from build123d import *

# Parameters (mm, degrees)
BOSS_EXTRUDE1_DEPTH = 12
SKETCH3_R           = 3.495
CUT_EXTRUDE2_DEPTH  = 78.961272437
CHAMFER1_SIZE       = 5


with BuildPart() as part:
    # Sketch1 → Boss-Extrude1 (new body)
    with BuildSketch(Plane.XY):
        Polygon((0, 0), (0, 58.6), (-35, 58.6), (-26.195973182, 49.795973182), (-26.195973182, 11.1), (-50, 0), align=None)
    extrude(amount=BOSS_EXTRUDE1_DEPTH)

    # Sketch3 → Cut-Extrude2 (cut, through all)
    with BuildSketch(Plane.XY.offset(12)):
        with Locations((-13.556619589, 25.36)):
            Circle(SKETCH3_R)
    extrude(amount=-CUT_EXTRUDE2_DEPTH, mode=Mode.SUBTRACT)

    # Chamfer1
    chamfer1_edges = [part.edges().sort_by_distance(p)[0] for p in [
        (0, 58.6, 6),
    ]]
    chamfer(chamfer1_edges, length=CHAMFER1_SIZE)


solid = part.part
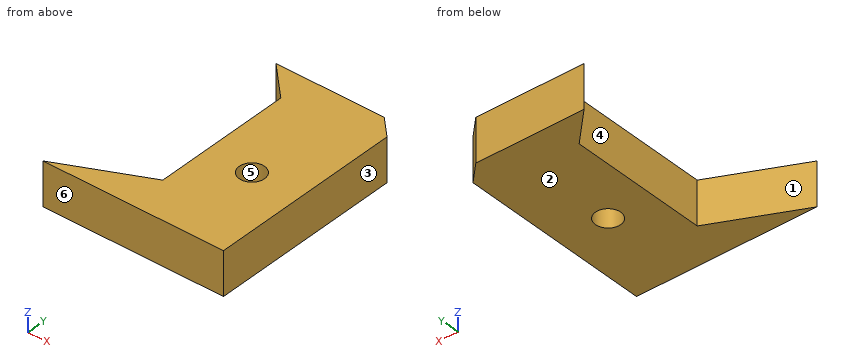
Geometry check sheet. Reference: the model listing, model coordinates, mm. Face numbers are marked on the shaded views. A direction names the side the tool comes from. Coordinates: 2 decimals unless noted, no trailing zeros. Order: outer loops, then holes, each group sorted by start corner. A loop starts at its lowest first (then second) coordinate and runs counter-clockwise, first axis right, second up. Notation, with made-up numbers: (23.25, -5) -> (71.25, -5) arc R27 cw to (71.25, 14) -> close; hole circle Ø11 at (40, 24.25). An arc over 180 degrees is marked (long way). Use a Markdown table: item, result. Add a question column.
1. Set-up check for the marked faces 1 and 2: record each of +Z, -Z, +X, -X, +Y, -Y from which the full face is reachable in a straight line by a thin tool's end or side.
2. Go/stop test with a flat-tipped pin: pin 1 Ø8 at (x, y) = (-13, 36.5) entering from -Z. Record where the tip stops, or that it passes through.
3. Mould release check, pull along X, two halves, no side actions. Record for the marked faces 3, 4, 5 and 6: pulls with the +X half, pulls with the -X half, needs draft (parallel to the pull), parting line crosses it, or undercut.
4. Cross-section at A-A (y = 25.36). Enter the section's corners in (x, z), and give its area (3 significant figures).
5. Cross-section at C-C (x = -3). Enter the section's corners in (y, z), and give its area (3 significant figures).
6. Material ranges on L1, parallel to X at y = 39, z = 9; L2, parallel to Y at x = -28, z = 7.5; L3, parallel to Y at x = -16, z = 6.25, recorded low to high.
7. Cross-section at D-D (y = 7). Enter the section's corners in (x, z).
8. Cross-section at B-B (z = 7). Enter the section's corners in (x, y) (3 decimals), and give its area (3 significant figures).
Filled sheet:
| question | item | result |
|---|---|---|
| 1 | face 1 | +Z, -Z, -X |
| 1 | face 2 | -Z, +X, -X, +Y, -Y |
| 2 | pin 1 | z = 0 |
| 3 | face 3 | pulls with the +X half |
| 3 | face 4 | pulls with the -X half |
| 3 | face 5 | undercut |
| 3 | face 6 | needs draft |
| 4 | outline | (-26.2, 0) -> (-17.05, 0) -> (-17.05, 12) -> (-26.2, 12) -> close; (-10.06, 0) -> (0, 0) -> (0, 12) -> (-10.06, 12) -> close |
| 4 | area | 230 mm2 |
| 5 | outline | (0, 0) -> (56.6, 0) -> (56.6, 12) -> (0, 12) -> close |
| 5 | area | 679 mm2 |
| 6 | L1 | -26.2 to 0 |
| 6 | L2 | 0 to 10.26, 51.6 to 58.6 |
| 6 | L3 | 0 to 22.86, 27.86 to 58.6 |
| 7 | outline | (-34.99, 0) -> (0, 0) -> (0, 12) -> (-34.99, 12) -> close |
| 8 | outline | (-50, 0) -> (0, 0) -> (0, 53.6) -> (-5, 58.6) -> (-35, 58.6) -> (-26.196, 49.796) -> (-26.196, 11.1) -> close; hole circle Ø6.99 at (-13.557, 25.36) |
| 8 | area | 1,660 mm2 |
